Autodesk Inventor part; units mm, degrees
ref_plane "YZ Plane" through (0, 0, 0) normal (1, 0, 0) x (0, 1, 0)
ref_plane "XZ Plane" through (0, 0, 0) normal (0, 1, 0) x (-1, 0, 0)
ref_plane "XY Plane" through (0, 0, 0) normal (0, 0, 1) x (1, 0, 0)
sketch "Esquisse1" plane through (0, 0, 0) normal (0, 0, 1) x (1, 0, 0)
  line L0 (-8.7953, 10.6752) -> (-4.7953, 10.6752)
  line L1 (-4.7953, -13.3248) -> (-8.7953, -13.3248)
  line L2 (3.2047, -3.3248) -> (3.2047, 0.6752)
  line L3 (-16.7953, 0.6752) -> (-16.7953, -3.3248)
  line L4 (3.2047, 0.6752) -> (-4.7953, 0.6752)
  line L5 (-8.7953, 0.6752) -> (-16.7953, 0.6752)
  line L6 (-4.7953, 10.6752) -> (-4.7953, 0.6752)
  line L7 (-4.7953, -3.3248) -> (-4.7953, -13.3248)
  line L8 (-16.7953, -3.3248) -> (-8.7953, -3.3248)
  line L9 (-4.7953, -3.3248) -> (3.2047, -3.3248)
  line L10 (-8.7953, -13.3248) -> (-8.7953, -3.3248)
  line L11 (-8.7953, 0.6752) -> (-8.7953, 10.6752)
  line L12 (-8.7953, 0.6752) -> (-4.7953, -3.3248) construction
  line L13 (-8.7953, -3.3248) -> (-4.7953, 0.6752) construction
  circle A0 centre (-6.7953, -1.3248) radius 1
  dimension "d0" = 10
  dimension "d1" = 8
  dimension "d2" = 4
  dimension "d5" = 2
extrude "Extrusion2" add sketch "Esquisse1" along normal blind 1.6
fillet "Congé1" radius 2 12 edges at (-8.7953, 0.6752, 0.8) (-8.7953, -3.3248, 0.8) (-16.7953, -3.3248, 0.8) (-16.7953, 0.6752, 0.8) (-8.7953, 10.6752, 0.8) (-4.7953, 10.6752, 0.8) (-4.7953, 0.6752, 0.8) (3.2047, 0.6752, 0.8) (3.2047, -3.3248, 0.8) (-4.7953, -3.3248, 0.8) (-4.7953, -13.3248, 0.8) (-8.7953, -13.3248, 0.8)
sketch "Esquisse2" plane through (0, 0, 1.6) normal (0, 0, 1) x (1, 0, 0)
  circle A0 centre (-6.7953, -1.3248) radius 1 construction
  circle A1 centre (-6.7953, -1.3248) radius 3.6
  circle A2 centre (-6.7953, -1.3248) radius 2.4
  point P0 (0, 0)
  dimension "d8" = 1.2
  dimension "d9" = 7.2
extrude "Extrusion3" add sketch "Esquisse2" along normal blind 3
properties part number "CoronaArm"
Design review of the part built by this model. Coordinates are the model's own, in mm. A direction names the side the tool comes from. Round coordinates to 2 decimals unless told otherwise and drop trailing zeros. Write each loop counter-clockwise with the first axis right and the second up, starting at its lowest first coordinate (ties: lowest second). Pieces come first, ordered by that corner, then holes. Notation, with made-up numbers: (64.25, 80.25) -> (100.25, 80.25) arc R20 ccw to (100.25, 91.25) -> close; hole circle Ø9 at (48, 66). An arc over 180 degrees is marked (long way). One line per item, written item: value. Start each with the question number.
Q1. Add section C-C (y = 1.5). Give the boundary of the cut face in (x, z), then the cut area to 3 significant figures.
Q2. Add section D-D (x = -14.25). Give the boundary of the cut face in (y, z), then the cut area to 3 significant figures.
Q3. To check wall thickness, follow probe 1 along X at (y, z) = (-5.5, 0.3); probe 2 along Z at (x, y) = (0.25, -1.5); probe 3 along Y at (x, z) = (-5.25, 2.9). State the ranges of each line that lie inside material, in increasing order.
Q4. Tool access review of faces 4 (the face through (-7.58, 2.19, 3.08)), 5 (the face through (-1, -3.325, 1)), 6 (the face through (-13, 0.675, 1)), 7 (the face through (-4.795, 6, 1)): name each direction out of +Z, -Z, +X, -X, +Y, -Y from which nothing blocks a thin tool from reaching the whole face with its end or side.
Q5. Add section A-A (x = -6.25). Give the boundary of the cut face in (y, z).
Q6. The part is to be moulded in two halves that separate along Y. For faces 1 (the face through (-1, 0.675, 1)), 2 (the face through (-4.506, -2.046, 3.079)), 3 (the face through (-8.795, 6, 1)), say which applies: pulls with the +Y half, pulls with the -Y half, needs draft (parallel to the pull), parting line crosses it, or undercut.
Q7. Insertion check: P1, Ø0.5, axis at y = -8.5, z = 0.5, coming from the +X side; P2, Ø1.6, axis at x = -6.8, y = -1.32, coming from the +Z side; P3, Ø0.5, axis at x = -1.5, z = 1, coming from the +Y side; P4, Ø2.5, axis at x = -7, y = -2, coming from the +Z side. Each pin has a flat end and moves straight along its axis. Give the tip position at first contact, or say it passes through.
Response:
1. outline: (-9.18, 0) -> (-4.41, 0) -> (-4.41, 1.6) -> (-4.56, 1.6) -> (-4.56, 4.6) -> (-9.03, 4.6) -> (-9.03, 1.6) -> (-9.18, 1.6) -> close
1. area: 21.0 mm^2
2. outline: (-3.32, 0) -> (0.68, 0) -> (0.68, 1.6) -> (-3.32, 1.6) -> close
2. area: 6.40 mm^2
3. probe 1: x = -8.8 to -4.8
3. probe 2: z = 0 to 1.6
3. probe 3: y = -4.58 to -3.16, 0.51 to 1.93
4. face 4: +Z
4. face 5: +Z, -Z, +X, -Y
4. face 6: +Z, -Z, -X, +Y
4. face 7: +Z, -Z, +X, +Y
5. outline: (-13.25, 0) -> (-2.16, 0) -> (-2.16, 1.6) -> (-3.66, 1.6) -> (-3.66, 4.6) -> (-4.88, 4.6) -> (-4.88, 1.6) -> (-13.25, 1.6) -> close; (-0.49, 0) -> (10.6, 0) -> (10.6, 1.6) -> (2.23, 1.6) -> (2.23, 4.6) -> (1.01, 4.6) -> (1.01, 1.6) -> (-0.49, 1.6) -> close
6. face 1: pulls with the +Y half
6. face 2: undercut
6. face 3: needs draft
7. P1: stops at x = -4.8
7. P2: passes through
7. P3: stops at y = 0.68
7. P4: stops at z = 1.6
